Could you check a few things on this model? Use its own coordinates, in mm. Give positions to 0.01 mm unless a question says otherwise; leave off trailing zeros. Loops run counter-clockwise (first coordinate to the right, second up) from the corner with the lowest first, then second, coordinate; pieces in that order, holes last.
1. Imagine slicing it at B-B (z = 1.8). List the corners of the cut face in (x, y) for me, plus the area to 3 significant figures.
2. Imagine slicing it at A-A (x = 0). List the corners of the cut face in (y, z) for me, plus the area to 3 significant figures.
3. Imagine slicing it at C-C (y = 11). List the corners of the cut face in (x, z) for me, plus the area to 3 significant figures.
4. I need wall thicknesses on line 1 along Y through (x, z) = (0, 2.25); line 2 along X through (y, z) = (-11, 2.05); line 3 along Y through (x, z) = (-1, 2.2). Which ranges of each line are inside material? Lowest first, please.
5. Thinking about a two-plate mould opening in Y: for faces 1 (the cylindrical face through (9.4, -14.43, 2.79)), 2 (the cylindrical face through (0.07, 12.6, 2.79)), 3 (the flat face through (10, 0, 3)), which applies, +Y half, -Y half, draft (parallel to the pull), parting line (faces both ways), or undercut?
Solid Edge part; units mm, degrees
sketch "Sketch1" plane through (0, 0, 0) normal (0, 0, 1) x (1, 0, 0)
  line L0 (10, -15) -> (-10, -15)
  line L1 (-10, -15) -> (-10, 15)
  line L2 (-10, 15) -> (10, 15)
  line L3 (10, 15) -> (10, -15)
  dimension "D1" = 10
  dimension "D2" = 10
extrude "Protrusion1" add sketch "Sketch1" along normal blind 5.5
hole "Hole_1" at (0, 11, 5.5) direction (0, 0, -1) diameter 3.2 end up to next
hole "Hole1" at (0, -11, 5.5) direction (0, 0, -1) diameter 3.2 end up to next
fillet "Round_1" radius 2 4 edges at (-10, -15, 2.75) (10, -15, 2.75) (-10, 15, 2.75) (10, 15, 2.75)
properties material "木材, アッシュ"
Derived:
1. outline: (-10, -13) arc R2 ccw to (-8, -15) - (8, -15) arc R2 ccw to (10, -13) - (10, 13) arc R2 ccw to (8, 15) - (-8, 15) arc R2 ccw to (-10, 13) - close; hole circle Ø3.2 at (0, -11); hole circle Ø3.2 at (0, 11)
1. area: 580 mm2
2. outline: (-15, 0) - (-12.6, 0) - (-12.6, 5.5) - (-15, 5.5) - close; (-9.4, 0) - (9.4, 0) - (9.4, 5.5) - (-9.4, 5.5) - close; (12.6, 0) - (15, 0) - (15, 5.5) - (12.6, 5.5) - close
2. area: 130 mm2
3. outline: (-10, 0) - (-1.6, 0) - (-1.6, 5.5) - (-10, 5.5) - close; (1.6, 0) - (10, 0) - (10, 5.5) - (1.6, 5.5) - close
3. area: 92.4 mm2
4. line 1: y = -15 to -12.6, -9.4 to 9.4, 12.6 to 15
4. line 2: x = -10 to -1.6, 1.6 to 10
4. line 3: y = -15 to -12.25, -9.75 to 9.75, 12.25 to 15
5. face 1: -Y half
5. face 2: undercut
5. face 3: draft
